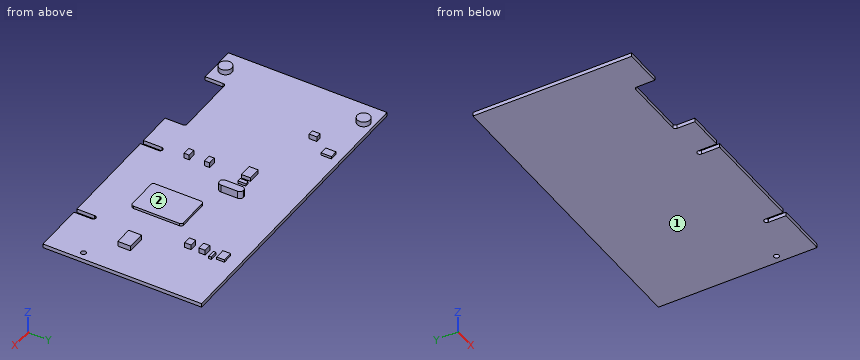
```python
from build123d import *

# Parameters (mm, degrees)
F0_W      = 120
F0_H      = 62
F1_DEPTH  = 1.5
F3_DEPTH  = 1.501
F5_DEPTH  = 1.501
F7_DEPTH  = 1.501
F8_R      = 1
F9_DEPTH  = 1.501
F10_W     = 7
F10_H     = 5
F11_DEPTH = 2
F13_DEPTH = 1
F14_W     = 3
F14_H     = 2.5
F15_DEPTH = 2
F16_W     = 3
F16_H     = 2.5
F17_DEPTH = 2
F18_W     = 3
F18_H     = 1
F19_DEPTH = 1
F20_W     = 4
F20_H     = 3
F21_DEPTH = 1
F23_DEPTH = 3
F24_W     = 1.5
F24_H     = 3
F25_DEPTH = 1
F26_W     = 5
F26_H     = 3.5
F27_DEPTH = 1.5
F28_W     = 3
F28_H     = 2
F29_DEPTH = 2
F30_W     = 3
F30_H     = 2
F31_DEPTH = 2
F32_R     = 2.5
F33_DEPTH = 2
F34_R     = 2.5
F35_DEPTH = 2
F36_W     = 3
F36_H     = 4
F37_DEPTH = 1
F38_W     = 2
F38_H     = 3
F39_DEPTH = 2


with BuildPart() as f1:
    # F0 (on Top) → F1 (new body)
    with BuildSketch(Plane.XY):
        with Locations((-1.138048, 13.651166)):
            Rectangle(F0_W, F0_H)
    extrude(amount=F1_DEPTH)

    # F2 (on face) → F3 (cut, through all)
    with BuildSketch(Plane.XY.offset(1.5)):
        with BuildLine():
            Line((-46.138048, -10.348834), (-46.138048, -17.348834))
            Line((-46.138048, -17.348834), (-20.138048, -17.348834))
            Line((-20.138048, -17.348834), (-20.138048, -10.348834))
            ThreePointArc((-20.138048, -10.348834), (-20.430941, -9.641727), (-21.138048, -9.348834))
            Line((-21.138048, -9.348834), (-45.138048, -9.348834))
            ThreePointArc((-45.138048, -9.348834), (-45.845155, -9.641727), (-46.138048, -10.348834))
        make_face()
    extrude(amount=-F3_DEPTH, mode=Mode.SUBTRACT)

    # F4 (on face) → F5 (cut, through all)
    with BuildSketch(Plane.XY.offset(1.5)):
        with BuildLine():
            Line((-6.138048, -10.157242), (-6.138048, -17.348834))
            Line((-6.138048, -17.348834), (-4.138048, -17.348834))
            Line((-4.138048, -17.348834), (-4.138048, -10.157242))
            ThreePointArc((-4.138048, -10.157242), (-5.138048, -9.157242), (-6.138048, -10.157242))
        make_face()
    extrude(amount=-F5_DEPTH, mode=Mode.SUBTRACT)

    # F6 (on face) → F7 (cut, through all)
    with BuildSketch(Plane.XY.offset(1.5)):
        with BuildLine():
            ThreePointArc((38.861952, -10.467094), (38.868969, -10.348834), (38.861952, -10.230573))
            Line((38.861952, -10.230573), (38.861952, -10.467094))
        make_face()
        with BuildLine():
            Line((36.875528, -10.463178), (36.875987, -10.230573))
            ThreePointArc((36.875987, -10.230573), (36.868971, -10.346862), (36.875528, -10.463178))
        make_face()
        with BuildLine():
            Line((38.861952, -10.467094), (38.861952, -10.230573))
            ThreePointArc((38.861952, -10.230573), (37.868969, -9.348834), (36.875987, -10.230573))
            Line((36.875987, -10.230573), (36.875528, -10.463178))
            Line((36.875528, -10.463178), (36.861952, -17.348834))
            Line((36.861952, -17.348834), (38.861952, -17.348834))
            Line((38.861952, -17.348834), (38.861952, -10.467094))
        make_face()
    extrude(amount=-F7_DEPTH, mode=Mode.SUBTRACT)

    # F8 (on face) → F9 (cut, through all)
    with BuildSketch(Plane.XY.offset(1.5)):
        with Locations((55.861952, -3.348834)):
            Circle(F8_R)
    extrude(amount=-F9_DEPTH, mode=Mode.SUBTRACT)

    # F10 (on face) → F11 (join)
    with BuildSketch(Plane.XY.offset(1.5)):
        with Locations((43.361952, 7.151166)):
            Rectangle(F10_W, F10_H)
    extrude(amount=F11_DEPTH)

    # F12 (on face) → F13 (join)
    with BuildSketch(Plane.XY.offset(1.5)):
        with BuildLine():
            Line((25.861952, 17.651166), (13.861952, 17.651166))
            ThreePointArc((13.861952, 17.651166), (13.154845, 17.358273), (12.861952, 16.651166))
            Line((12.861952, 16.651166), (12.861952, -1.348834))
            ThreePointArc((12.861952, -1.348834), (13.154845, -2.05594), (13.861952, -2.348834))
            Line((13.861952, -2.348834), (25.861952, -2.348834))
            ThreePointArc((25.861952, -2.348834), (26.569059, -2.05594), (26.861952, -1.348834))
            Line((26.861952, -1.348834), (26.861952, 16.651166))
            ThreePointArc((26.861952, 16.651166), (26.569059, 17.358273), (25.861952, 17.651166))
        make_face()
    extrude(amount=F13_DEPTH)

    # F14 (on face) → F15 (join)
    with BuildSketch(Plane.XY.offset(1.5)):
        with Locations((34.361952, 25.401166)):
            Rectangle(F14_W, F14_H)
    extrude(amount=F15_DEPTH)

    # F16 (on face) → F17 (join)
    with BuildSketch(Plane.XY.offset(1.5)):
        with Locations((34.361952, 30.901166)):
            Rectangle(F16_W, F16_H)
    extrude(amount=F17_DEPTH)

    # F18 (on face) → F19 (join)
    with BuildSketch(Plane.XY.offset(1.5)):
        with Locations((35.361952, 34.651166)):
            Rectangle(F18_W, F18_H)
    extrude(amount=F19_DEPTH)

    # F20 (on face) → F21 (join)
    with BuildSketch(Plane.XY.offset(1.5)):
        with Locations((33.861952, 38.151166)):
            Rectangle(F20_W, F20_H)
    extrude(amount=F21_DEPTH)

    # F22 (on face) → F23 (join)
    with BuildSketch(Plane.XY.offset(1.5)):
        with BuildLine():
            ThreePointArc((2.654845, 27.151166), (1.594185, 26.711826), (1.154845, 25.651166))
            Line((1.154845, 25.651166), (1.154845, 19.151166))
            ThreePointArc((1.154845, 19.151166), (1.594185, 18.090506), (2.654845, 17.651166))
            ThreePointArc((2.654845, 17.651166), (3.715505, 18.090506), (4.154845, 19.151166))
            Line((4.154845, 19.151166), (4.154845, 25.651166))
            ThreePointArc((4.154845, 25.651166), (3.715505, 26.711826), (2.654845, 27.151166))
        make_face()
    extrude(amount=F23_DEPTH)

    # F24 (on face) → F25 (join)
    with BuildSketch(Plane.XY.offset(1.5)):
        with Locations((-3.595155, 23.151166)):
            Rectangle(F24_W, F24_H)
    extrude(amount=F25_DEPTH)

    # F26 (on face) → F27 (join)
    with BuildSketch(Plane.XY.offset(1.5)):
        with Locations((-8.345155, 22.901166)):
            Rectangle(F26_W, F26_H)
    extrude(amount=F27_DEPTH)

    # F28 (on face) → F29 (join)
    with BuildSketch(Plane.XY.offset(1.5)):
        with Locations((-6.638048, 8.151166)):
            Rectangle(F28_W, F28_H)
    extrude(amount=F29_DEPTH)

    # F30 (on face) → F31 (join)
    with BuildSketch(Plane.XY.offset(1.5)):
        with Locations((-6.638048, 0.151166)):
            Rectangle(F30_W, F30_H)
    extrude(amount=F31_DEPTH)

    # F32 (on face) → F33 (join)
    with BuildSketch(Plane.XY.offset(1.5)):
        with Locations((-52.638048, 40.651166)):
            Circle(F32_R)
    extrude(amount=F33_DEPTH)

    # F34 (on face) → F35 (join)
    with BuildSketch(Plane.XY.offset(1.5)):
        with Locations((-52.638048, -13.348834)):
            Circle(F34_R)
    extrude(amount=F35_DEPTH)

    # F36 (on face) → F37 (join)
    with BuildSketch(Plane.XY.offset(1.5)):
        with Locations((-31.638048, 39.651166)):
            Rectangle(F36_W, F36_H)
    extrude(amount=F37_DEPTH)

    # F38 (on face) → F39 (join)
    with BuildSketch(Plane.XY.offset(1.5)):
        with Locations((-36.638048, 31.151166)):
            Rectangle(F38_W, F38_H)
    extrude(amount=F39_DEPTH)


solid = f1.part
```
For this review, take the finished solid that the model builds, in its own axes (mm). Face numbers are marked on the shaded views. A direction names the side the tool comes from. Coordinates: 2 decimals unless noted, no trailing zeros. Write each loop counter-clockwise with the first axis right and the second up, starting at its lowest first coordinate (ties: lowest second). Pieces come first, ordered by that corner, then holes. Notation, with made-up numbers: (37, 79.5) - (82, 79.5) arc R23 ccw to (82, 87.5) - close; hole circle Ø5 at (76, 8). An arc over 180 degrees is marked (long way). Put each result on its own line as item: value.
1. Add section C-C, the plane y = 23. Give the boundary of the cut face in (x, z).
Values found:
outline: (-61.14, 0) - (58.86, 0) - (58.86, 1.5) - (4.15, 1.5) - (4.15, 4.5) - (1.15, 4.5) - (1.15, 1.5) - (-2.85, 1.5) - (-2.85, 2.5) - (-4.35, 2.5) - (-4.35, 1.5) - (-5.85, 1.5) - (-5.85, 3) - (-10.85, 3) - (-10.85, 1.5) - (-61.14, 1.5) - close
2. Add section A-A, the plane z = 0.75. Give the boundary of the cut face in (x, y).
Values found:
outline: (-61.14, -17.35) - (-46.14, -17.35) - (-46.14, -10.35) arc R1 cw to (-45.14, -9.35) - (-21.14, -9.35) arc R1 cw to (-20.14, -10.35) - (-20.14, -17.35) - (-6.14, -17.35) - (-6.14, -10.16) arc R1 cw to (-4.14, -10.16) - (-4.14, -17.35) - (36.86, -17.35) - (36.88, -10.46) arc R1 cw to (36.88, -10.23) arc R1 cw to (38.86, -10.23) arc R1 cw to (38.86, -10.47) - (38.86, -17.35) - (58.86, -17.35) - (58.86, 44.65) - (-61.14, 44.65) - close; hole circle Ø2 at (55.86, -3.35)
3. For pin 1 (0.6 mm diameter, centred on x = -7.5, y = 0.5, fed in from +Z); pin 2 (0.8 mm diameter, centred on x = 33.5, z = 2, fed in from +Y); pin 3 (1.6 mm diameter, centred on y = 30.5, z = 2.5, fed in from +X), all flat-tipped, find the tip position at first contact; note any pin that passes through.
Values found:
pin 1: z = 3.5
pin 2: y = 39.65
pin 3: x = 35.86
4. Wall thickness on probe 1 along Z at (x, y) = (51.5, 38); probe 2 along X at (y, z) = (19.5, 2.7); probe 3 along Z at (x, y) = (17.5, 13.5): over which ranges is each line inside the solid? List them lowest first.
Values found:
probe 1: 0 to 1.5
probe 2: 1.15 to 4.15
probe 3: 0 to 2.5
5. Machinability: for the marked faces 1 and 2, which of the approach directions +Z, -Z, +X, -X, +Y, -Y give a long, thin tool a straight path to every point of the face, cutting with its end or side? Answer none if there is none.
Values found:
face 1: -Z, +X, -X, +Y, -Y
face 2: +Z, +Y, -Y
6. Add section B-B, the plane x = 44.5. Give the boundary of the cut face in (y, z), then the cut area to 3 significant figures.
Values found:
outline: (-17.35, 0) - (44.65, 0) - (44.65, 1.5) - (9.65, 1.5) - (9.65, 3.5) - (4.65, 3.5) - (4.65, 1.5) - (-17.35, 1.5) - close
area: 103 mm²
7. Add section D-D, the plane x = 21.5. Give the boundary of the cut face in (y, z).
Values found:
outline: (-17.35, 0) - (44.65, 0) - (44.65, 1.5) - (17.65, 1.5) - (17.65, 2.5) - (-2.35, 2.5) - (-2.35, 1.5) - (-17.35, 1.5) - close
